Could you check a few things on this model? Use its own coordinates, in mm. A direction names the side the tool comes from. Round coordinates to 2 decimals unless told otherwise and drop trailing zeros. Loops run counter-clockwise (first coordinate to the right, second up) from the corner with the lowest first, then second, coordinate; pieces in that order, holes last.
from build123d import *

# Parameters (mm, degrees)
F0_R          = 6
F1_DEPTH      = 10
F2_R          = 10
F3_DEPTH      = 8
F3_DEPTH_BACK = 8


with BuildPart() as f1:
    # F0 (on Top) → F1 (new body)
    with BuildSketch(Plane.XY):
        with BuildLine():
            ThreePointArc((50.720724, 17.985565), (30.362055, 23.224109), (13.956018, 36.367918))
            ThreePointArc((13.956018, 36.367918), (-6.032896, 41.958896), (-18, 25))
            Line((-18, 25), (-18, -25))
            ThreePointArc((-18, -25), (-6.032896, -41.958896), (13.956018, -36.367918))
            ThreePointArc((13.956018, -36.367918), (30.362055, -23.224109), (50.720724, -17.985565))
            ThreePointArc((50.720724, -17.985565), (68, 0), (50.720724, 17.985565))
        make_face()
        with Locations((0, -25)):
            Circle(F0_R, mode=Mode.SUBTRACT)
        with Locations((0, 25)):
            Circle(F0_R, mode=Mode.SUBTRACT)
        with Locations((50, 0)):
            Circle(F0_R, mode=Mode.SUBTRACT)
    extrude(amount=F1_DEPTH)

    # F2 (on Front) → F3 (join, two sides)
    with BuildSketch(Plane.XZ) as f3_sk:
        with BuildLine():
            ThreePointArc((33.633398, 10), (-8.875104, 17.449895), (-46.316665, 38.911565))
            ThreePointArc((-46.316665, 38.911565), (-81.076694, 29.481496), (-60.387876, 0))
            Line((-60.387876, 0), (33.633398, 0))
            Line((33.633398, 0), (33.633398, 10))
        make_face()
        with Locations((-60.387876, 22)):
            Circle(F2_R, mode=Mode.SUBTRACT)
    extrude(amount=F3_DEPTH)
    extrude(f3_sk.sketch, amount=-F3_DEPTH_BACK)


solid = f1.part
Item 1: If we section it at A-A, the plane y = 0: Please give me the cut outline in (x, z).
Results list:
outline: (-60.39, 0) - (44, 0) - (44, 10) - (33.63, 10) arc R125 cw to (-46.32, 38.91) arc R22 ccw (long way) to start; (56, 0) - (68, 0) - (68, 10) - (56, 10) - close; hole circle Ø20 at (-60.39, 22)
Item 2: If we section it at C-C, the plane x = 0: Please give me the cut outline in (y, z), then the cut area to 3 significant figures.
Results list:
outline: (-43, 0) - (-31, 0) - (-31, 10) - (-43, 10) - close; (-19, 0) - (19, 0) - (19, 10) - (8, 10) - (8, 14.61) - (-8, 14.61) - (-8, 10) - (-19, 10) - close; (31, 0) - (43, 0) - (43, 10) - (31, 10) - close
area: 694 mm2
Item 3: If I drill on line 1 along Y through (x, z) = (0, 2); line 2 along Y through (x, z) = (4, 6.5); line 3 along Z through (x, y) = (55.5, 8), over which ranges is the centre line in solid material (lowest first)?
Results list:
line 1: y = -43 to -31, -19 to 19, 31 to 43
line 2: y = -42.55 to -29.47, -20.53 to 20.53, 29.47 to 42.55
line 3: z = 0 to 10
Item 4: If we section it at B-B, the plane z = 19.5: Please give me the cut outline in (x, y).
Results list:
outline: (-82.25, -8) - (-70.07, -8) - (-70.07, 8) - (-82.25, 8) - close; (-50.71, -8) - (-14.17, -8) - (-14.17, 8) - (-50.71, 8) - close
Item 5: For faces 1 (the flat face through (-18, 17, 5)), 2 (the flat face through (-18, -16, 5)), 3 (the cylindrical face through (-1.301, 19.143, 4.93)), which set-ups out of +Z, -Z, +X, -X, +Y, -Y let a thin tool reach every point of the face, with its end or its side?
Results list:
face 1: +Z, -Z, -X, +Y
face 2: +Z, -Z, -X, -Y
face 3: +Z, -Z
Item 6: Will these pins go through, and if not, where does the flat tip stop? pin 1 (6 mm diameter, centred on x = 41.5, y = 23, fed in from -Z); pin 2 (8 mm diameter, centred on y = 3, z = 33, fed in from -X); pin 3 (5 mm diameter, centred on y = 7, z = 38.5, fed in from +X); pin 4 (11 mm diameter, centred on y = -19.5, z = 2.5, fed in from -X).
Results list:
pin 1: passes through
pin 2: stops at x = -81.24
pin 3: stops at x = -42.68
pin 4: stops at x = -18
Item 7: If we section it at D-D, the plane z = 28: Please give me the cut outline in (x, y).
Results list:
outline: (-81.55, -8) - (-68.39, -8) - (-68.39, 8) - (-81.55, 8) - close; (-52.39, -8) - (-30.99, -8) - (-30.99, 8) - (-52.39, 8) - close
Item 8: We'd pull the mould along Z, two halves only. Please class faces 4 (the cylindrical face through (-50.85, 0.11, 25)), 5 (the cylindrical face through (68, 0, 5)), 6 (the cylindrical face through (-8.304, -0.112, 17.245)), 7 (the cylindrical face through (-80.87, -0.11, 30.03)): released by +Z, released by -Z, zero draft, split by the parting line, or undercut.
Results list:
face 4: undercut
face 5: zero draft
face 6: released by +Z
face 7: split by the parting line
